from build123d import *

# Parameters (mm, degrees)
SKETCH1_W                                       = 125.999061968
SKETCH1_H                                       = 101.6
SKETCH1_R                                       = 3.45
SKETCH1_R_2                                     = 1.27
BOSS_EXTRUDE1_DEPTH                             = 60.325
SKETCH1_3_W                                     = 9.525
SKETCH1_3_H                                     = 20
BOSS_EXTRUDE2_DEPTH                             = 25
CUT_EXTRUDE1_DEPTH                              = 149.645582651
CUT_EXTRUDE1_DEPTH_BACK                         = 149.645582651
SKETCH2_R                                       = 1.5999968
CSK_FOR_8_FLAT_HEAD_MACHINE_SCREW_2_COUNT       = 2
CSK_FOR_8_FLAT_HEAD_MACHINE_SCREW_2_PITCH       = 38.1
CSK_FOR_8_FLAT_HEAD_MACHINE_SCREW_3_COUNT       = 2
CSK_FOR_8_FLAT_HEAD_MACHINE_SCREW_3_PITCH       = 84.060186176
CSK_FOR_8_FLAT_HEAD_MACHINE_SCREW_4_COUNT       = 2
CSK_FOR_8_FLAT_HEAD_MACHINE_SCREW_4_PITCH       = 74.93
CSK_FOR_M3_FLAT_HEAD_MACHINE_SCREW1_D           = 3.4
CSK_FOR_M3_FLAT_HEAD_MACHINE_SCREW1_CSINK_D     = 6.7
CSK_FOR_M3_FLAT_HEAD_MACHINE_SCREW1_CSINK_ANGLE = 90
CHAMFER1_SIZE                                   = 0.508
CHAMFER2_SIZE                                   = 1.905


with BuildPart() as part:
    # Sketch1 → Boss-Extrude1 (new body)
    with BuildSketch(Plane.XY):
        Rectangle(SKETCH1_W, SKETCH1_H)
        with Locations((-25.299530984, 34.925)):
            Circle(SKETCH1_R, mode=Mode.SUBTRACT)
        with Locations((-0.299530984, 34.925)):
            Circle(SKETCH1_R, mode=Mode.SUBTRACT)
        with Locations((21.455469016, 22.225)):
            Circle(SKETCH1_R_2, mode=Mode.SUBTRACT)
        with Locations((21.455469016, -15.875)):
            Circle(SKETCH1_R_2, mode=Mode.SUBTRACT)
        with Locations((-53.474530984, -15.875)):
            Circle(SKETCH1_R_2, mode=Mode.SUBTRACT)
        with Locations((-53.474530984, 22.225)):
            Circle(SKETCH1_R_2, mode=Mode.SUBTRACT)
    extrude(amount=-BOSS_EXTRUDE1_DEPTH)

    # Sketch1_3 → Boss-Extrude2 (add)
    with BuildSketch(Plane.XY):
        with Locations((37.962030984, -40.8)):
            Rectangle(SKETCH1_3_W, SKETCH1_3_H)
        with Locations((58.237030984, -40.8)):
            Rectangle(SKETCH1_3_W, SKETCH1_3_H)
    extrude(amount=BOSS_EXTRUDE2_DEPTH)

    # Sketch2 → Cut-Extrude1 (cut, two sides: drawn at the far end of the back side and taken through both)
    with BuildSketch(Plane(origin=(62.999530984, 0, 0), x_dir=(0, 0, -1), z_dir=(1, 0, 0)).offset(-CUT_EXTRUDE1_DEPTH_BACK)):
        with Locations(Location((-15, -40.8, 0), (0, 0, 180))):
            Circle(SKETCH2_R)
    extrude(amount=CUT_EXTRUDE1_DEPTH + CUT_EXTRUDE1_DEPTH_BACK, mode=Mode.SUBTRACT)

    # Sketch6 → CSK for _8 Flat Head Machine Screw _100 (revolve, cut)
    with BuildSketch(Plane(origin=(-53.474530984, 22.225, 0), x_dir=(0, -1, 0), z_dir=(1, 0, 0))):
        Polygon((0, 0), (0, 60.325), (2.2479, 60.325), (2.2479, 39.751763788), (4.216395428, 38.1), (4.216395428, 0), align=None)
    csk_for_8_flat_head_machine_screw_100 = revolve(axis=Axis((-53.474530984, 22.225, 6.35), (0, 0, -1)), mode=Mode.SUBTRACT)

    # CSK for _8 Flat Head Machine Screw _ 2: CSK for _8 Flat Head Machine Screw _100 ×2
    with Locations(*[(0, -i * CSK_FOR_8_FLAT_HEAD_MACHINE_SCREW_2_PITCH, 0) for i in range(1, CSK_FOR_8_FLAT_HEAD_MACHINE_SCREW_2_COUNT)]):
        add(csk_for_8_flat_head_machine_screw_100, mode=Mode.SUBTRACT)

    # CSK for _8 Flat Head Machine Screw _ 3: CSK for _8 Flat Head Machine Screw _100 ×2
    with Locations(*[Vector(0.8913851302068038, -0.453246676376341, 0) * (i * CSK_FOR_8_FLAT_HEAD_MACHINE_SCREW_3_PITCH) for i in range(1, CSK_FOR_8_FLAT_HEAD_MACHINE_SCREW_3_COUNT)]):
        add(csk_for_8_flat_head_machine_screw_100, mode=Mode.SUBTRACT)

    # CSK for _8 Flat Head Machine Screw _ 4: CSK for _8 Flat Head Machine Screw _100 ×2
    with Locations(*[(i * CSK_FOR_8_FLAT_HEAD_MACHINE_SCREW_4_PITCH, 0, 0) for i in range(1, CSK_FOR_8_FLAT_HEAD_MACHINE_SCREW_4_COUNT)]):
        add(csk_for_8_flat_head_machine_screw_100, mode=Mode.SUBTRACT)

    # CSK for M3 Flat Head Machine Screw1 (through all)
    with Locations(Plane(origin=(62.999530984, 0, 0), x_dir=(0, 0, -1), z_dir=(1, 0, 0))):
        with Locations((-15, -40.8)):
            CounterSinkHole(CSK_FOR_M3_FLAT_HEAD_MACHINE_SCREW1_D / 2, CSK_FOR_M3_FLAT_HEAD_MACHINE_SCREW1_CSINK_D / 2, counter_sink_angle=CSK_FOR_M3_FLAT_HEAD_MACHINE_SCREW1_CSINK_ANGLE)

    # Chamfer1
    chamfer1_edges = [part.edges().sort_by_distance(p)[0] for p in [
        (-53.474530984, 26.441395428, 0),
        (-28.749530984, 34.925, 0),
        (-3.749530984, 34.925, 0),
        (21.455469016, 26.441395428, 0),
        (21.455469016, -11.658604572, 0),
        (-53.474530984, -11.658604572, 0),
    ]]
    chamfer(chamfer1_edges, length=CHAMFER1_SIZE)

    # Chamfer2
    chamfer2_edges = [part.edges().sort_by_distance(p)[0] for p in [
        (-14.9, -50.8, 0),
        (33.199530984, -40.8, 25),
        (33.199530984, -30.8, 12.5),
        (37.962030984, -50.8, 25),
        (33.199530984, -50.8, 12.5),
        (42.724530984, -40.8, 0),
        (42.724530984, -50.8, 12.5),
        (37.962030984, -30.8, 0),
        (42.724530984, -30.8, 12.5),
        (42.724530984, -40.8, 25),
        (37.962030984, -30.8, 25),
        (33.199530984, -40.8, 0),
        (0, 50.8, 0),
        (48.099530984, -50.8, 0),
        (53.474530984, -40.8, 25),
        (53.474530984, -30.8, 12.5),
        (58.237030984, -50.8, 25),
        (-62.999530984, 0, 0),
        (53.474530984, -50.8, 12.5),
        (62.999530984, -40.8, 25),
        (58.237030984, -30.8, 0),
        (62.999530984, -30.8, 12.5),
        (58.237030984, -30.8, 25),
        (53.474530984, -40.8, 0),
        (62.999530984, 10, 0),
        (62.999530984, 50.8, -30.1625),
        (-62.999530984, 50.8, -30.1625),
        (-62.999530984, -50.8, -30.1625),
        (62.999530984, -50.8, -17.6625),
    ]]
    chamfer(chamfer2_edges, length=CHAMFER2_SIZE)


solid = part.part
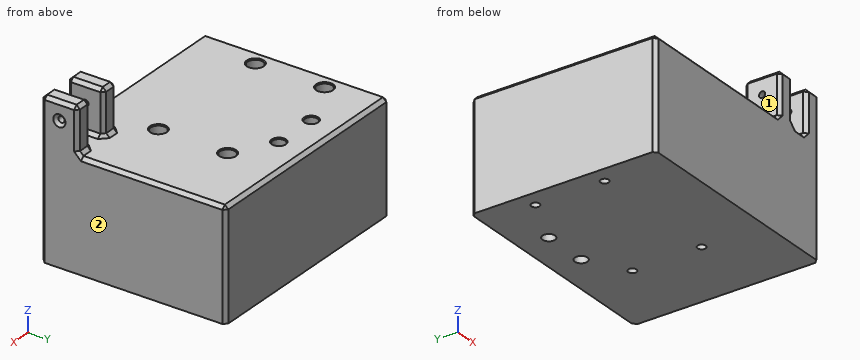
Model file for the job. Use its own axes, mm. Face numbers are marked on the shaded views. A direction names the side the tool comes from. Give positions to 0.01 mm unless a question says otherwise; leave off trailing zeros. Loops run counter-clockwise (first coordinate to the right, second up) from the corner with the lowest first, then second, coordinate; pieces in that order, holes last.
1) Saw through at A-A (y = -40.8). Write the cut outline in (x, z) (3 decimals).
2) Saw through at B-B (z = 15). Write the cut outline in (x, y) (3 decimals).
3) Tool access for the marked faces 1 and 2: list every direction of +Z, -Z, +X, -X, +Y, -Y with a clear straight run to the whole face (end or side of a thin tool).
4) Wall check: line 1 (Y direction, x = 38, z = 15); line 2 (Y direction, x = -52, z = -51); line 3 (Z direction, x = 16, y = -18) (3 decimals). Give the ranges that are in metal, low to high.
5) Flat gauge pins, fed straight in: pin 1 Ø8 at (x, y) = (-25.3, 34.92) entering from +Z; pin 2 Ø5 at (x, y) = (21.46, -15.87) entering from +Z; pin 3 Ø5 at (y, z) = (-43.5, 8) entering from -X; pin 4 Ø5 at (x, y) = (21.46, 22.22) entering from -Z (3 decimals). Where does each tip first touch, or does it go through?
6) Saw through at C-C (x = -42). Write the cut outline in (y, z) (3 decimals), plus the area to 3 significant figures.
7) Saw through at D-D (z = -17). Write the cut outline in (x, y) (3 decimals), plus the area to 3 significant figures.
Answer block:
1. outline: (-63, -60.325) - (63, -60.325) - (63, 11.65) - (61.35, 13.3) - (53.475, 13.3) - (53.475, 1.905) - (51.57, 0) - (44.63, 0) - (42.725, 1.905) - (42.725, 13.3) - (33.2, 13.3) - (33.2, 1.905) - (31.295, 0) - (-61.095, 0) - (-63, -1.905) - close; (33.2, 16.7) - (42.725, 16.7) - (42.725, 23.095) - (40.82, 25) - (35.105, 25) - (33.2, 23.095) - close; (53.475, 16.7) - (61.35, 16.7) - (63, 18.35) - (63, 23.095) - (61.095, 25) - (55.38, 25) - (53.475, 23.095) - close
2. outline: (33.2, -48.895) - (35.105, -50.8) - (40.82, -50.8) - (42.725, -48.895) - (42.725, -42.5) - (33.2, -42.5) - close; (33.2, -39.1) - (42.725, -39.1) - (42.725, -32.705) - (40.82, -30.8) - (35.105, -30.8) - (33.2, -32.705) - close; (53.475, -48.895) - (55.38, -50.8) - (61.095, -50.8) - (63, -48.895) - (63, -44.15) - (61.35, -42.5) - (53.475, -42.5) - close; (53.475, -39.1) - (61.35, -39.1) - (63, -37.45) - (63, -32.705) - (61.095, -30.8) - (55.38, -30.8) - (53.475, -32.705) - close
3. face 1: +Z, -X, +Y, -Y
3. face 2: +Z, -Z, +X, +Y, -Y
4. line 1: y = -50.8 to -42.5, -39.1 to -30.8
4. line 2: y = -50.8 to -17.57, -14.18 to 20.53, 23.92 to 50.8
4. line 3: z = -60.325 to 0
5. pin 1: stops at z = 0
5. pin 2: stops at z = -39.53
5. pin 3: stops at x = 33.2
5. pin 4: stops at z = -60.325
6. outline: (-50.8, -60.325) - (50.8, -60.325) - (50.8, -1.905) - (48.895, 0) - (-48.895, 0) - (-50.8, -1.905) - close
6. area: 6,130 mm2
7. outline: (-63, -48.895) - (-61.095, -50.8) - (61.095, -50.8) - (63, -48.895) - (63, 48.895) - (61.095, 50.8) - (-61.095, 50.8) - (-63, 48.895) - close; hole circle Ø8.433 at (-53.475, -15.875); hole circle Ø8.433 at (-53.475, 22.225); hole circle Ø6.9 at (-25.3, 34.925); hole circle Ø6.9 at (-0.3, 34.925); hole circle Ø8.433 at (21.455, -15.875); hole circle Ø8.433 at (21.455, 22.225)
7. area: 12,500 mm2
